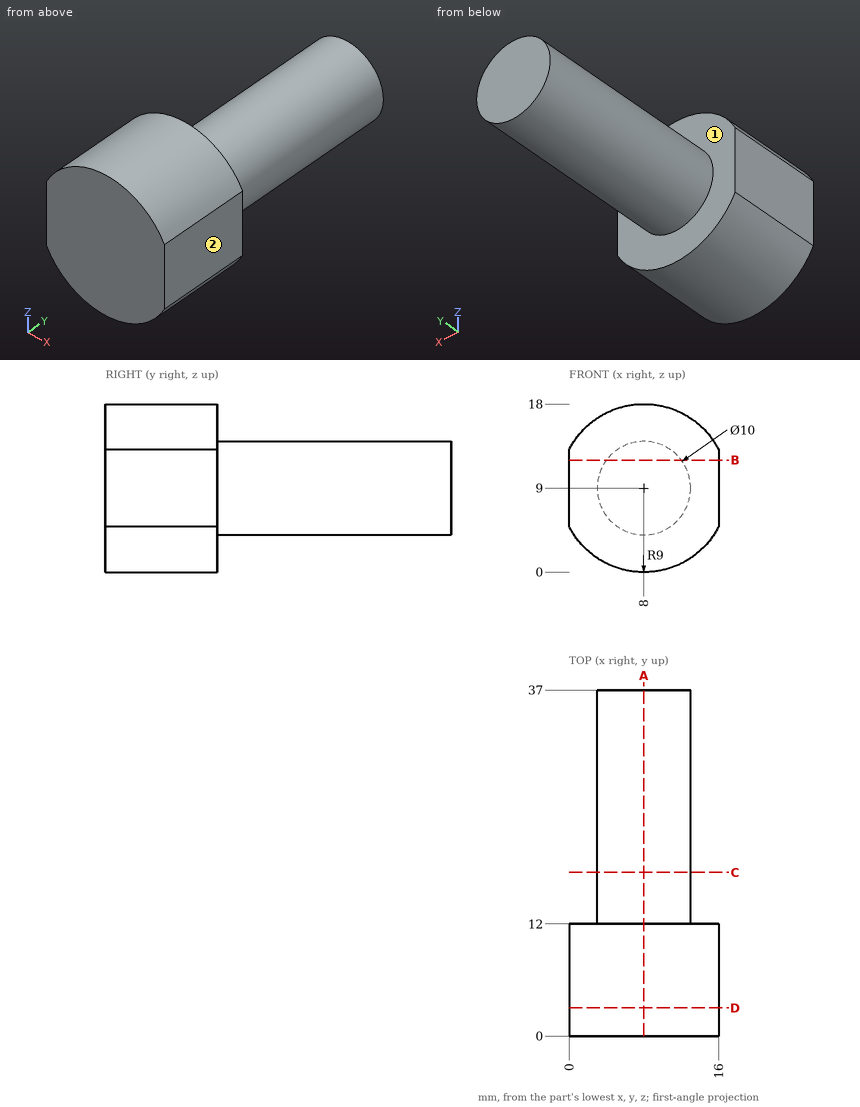
Source: three-view drawing plus pictorial views. Frame: mm from the lowest corner of the part. A direction names the side the tool comes from. Give positions to 0.01 mm unless a question says otherwise; leave off trailing zeros. Loops run counter-clockwise (first coordinate to the right, second up) from the corner with the lowest first, then second, coordinate; pieces in that order, holes last.
1) Section query B-B on z = 12. Return the cut outline in (x, y), and give its area (3 significant figures).
A:
outline: (0, 0) - (16, 0) - (16, 12) - (12, 12) - (12, 37) - (4, 37) - (4, 12) - (0, 12) - close
area: 392 mm2
2) Section query D-D on y = 3. Return the cut outline in (x, z).
A:
outline: (0, 4.88) arc R9 ccw to (16, 4.88) - (16, 13.12) arc R9 ccw to (0, 13.12) - close
3) Line query: L1, parallel to Y at x = 11.75, z = 3.75; L2, parallel to X at y = 25, z = 9.75; L3, parallel to Z at x = 8.25, y = 14. Output: solid intervals per line, ascending.
A:
L1: y = 0 to 12
L2: x = 3.06 to 12.94
L3: z = 4.01 to 13.99
4) Section query C-C on y = 17.5. Return the cut outline in (x, z), and give its area (3 significant figures).
A:
outline: circle Ø10 at (8, 9)
area: 78.5 mm2
5) Reachability of the marked faces 1 and 2 from +Z, -Z, +X, -X, +Y, -Y: full face, straight path, thin tool, end or side. Return the list, or none.
A:
face 1: +Y
face 2: +Z, -Z, +X, +Y, -Y
6) Contact query for flat-ended pins moving along their axis: pin 1 (8 mm diameter, centred on x = 4.5, y = 33, fed in from +Z); pin 2 (1 mm diameter, centred on y = 31.5, z = 11.5, fed in from -X); pin 3 (8 mm diameter, centred on x = 10, z = 3, fed in from +Y); pin 4 (3 mm diameter, centred on x = 12, y = 14.5, fed in from +Z). Output: stop coordinate, or through.
A:
pin 1: stops at z = 14
pin 2: stops at x = 3.42
pin 3: stops at y = 37
pin 4: stops at z = 13.33
7) Section query A-A on x = 8. Return the cut outline in (y, z).
A:
outline: (0, 0) - (12, 0) - (12, 4) - (37, 4) - (37, 14) - (12, 14) - (12, 18) - (0, 18) - close
